from build123d import *

# Parameters (mm, degrees)
BOSS_EXTRUDE1_DEPTH = 16
SKETCH2_R           = 4
CUT_EXTRUDE1_DEPTH  = 40
SKETCH3_W           = 26
SKETCH3_H           = 4
CUT_EXTRUDE2_DEPTH  = 40
SKETCH4_R           = 1.25
CUT_EXTRUDE3_DEPTH  = 40


with BuildPart() as part:
    # Sketch1 → Boss-Extrude1 (new body)
    with BuildSketch(Plane.XY):
        Polygon((0, 0), (32, 0), (32, 12), (26, 18), (6, 18), (0, 12), align=None)
    extrude(amount=BOSS_EXTRUDE1_DEPTH)

    # Sketch2 → Cut-Extrude1 (cut, symmetric)
    with BuildSketch(Plane(origin=(0, 0, 0), x_dir=(1, 0, 0), z_dir=(0, 1, 0))):
        with Locations(Location((11, -8, 0), (0, 0, 270))):
            Circle(SKETCH2_R)
        with Locations(Location((21, -8, 0), (0, 0, 270))):
            Circle(SKETCH2_R)
    extrude(amount=CUT_EXTRUDE1_DEPTH, both=True, mode=Mode.SUBTRACT)

    # Sketch3 → Cut-Extrude2 (cut, symmetric)
    with BuildSketch(Plane.XY):
        with Locations((13, 6)):
            Rectangle(SKETCH3_W, SKETCH3_H)
    extrude(amount=CUT_EXTRUDE2_DEPTH, both=True, mode=Mode.SUBTRACT)

    # Sketch4 → Cut-Extrude3 (cut, symmetric)
    with BuildSketch(Plane.XY):
        with Locations((29, 11)):
            Circle(SKETCH4_R)
    extrude(amount=CUT_EXTRUDE3_DEPTH, both=True, mode=Mode.SUBTRACT)


solid = part.part
Geometry: final body of the model. Coordinates: model frame, mm. A direction names the side the tool comes from. Round coordinates to 2 decimals unless told otherwise and drop trailing zeros. Order: outer loops, then holes, each group sorted by start corner. A loop starts at its lowest first (then second) coordinate and runs counter-clockwise, first axis right, second up. Notation, with made-up numbers: (77.25, 42.25) -> (111.25, 42.25) arc R18 ccw to (111.25, 65.25) -> close; hole circle Ø5 at (85, 35). An arc over 180 degrees is marked (long way). Put each result on its own line as item: value. Start each with the question number.
Q1. Line query: probe 1 along X at (y, z) = (2.8, 8); probe 2 along Y at (x, z) = (25.5, 13.5); probe 3 along Y at (x, z) = (29, 10.5). Output: solid intervals per line, ascending.
Q2. First-contact query: pin 1 (1.5 mm diameter, centred on x = 29, y = 11, fed in from +Z). Flat tip, straight axial feed; report the tip coordinate or a pass-through.
Q3. Section B-B on z = 8. Return the cut outline in (x, y), and give its area (3 significant figures).
Q4. Section D-D on x = 29. Return the cut outline in (y, z).
Q5. Section A-A on y = 11. Return the cut outline in (x, z), and give its area (3 significant figures).
Q6. Reachability of faces 5 (the flat face through (0, 2, 8)), 6 (the flat face through (26, 6, 8)) from +Z, -Z, +X, -X, +Y, -Y: full face, straight path, thin tool, end or side. Return the list, or none.
Q7. Section C-C on x = 21. Return the cut outline in (y, z).
Q8. Pull-direction query (Y, two-part tool) for faces 1 (the flat face through (13, 8, 12)), 2 (the flat face through (13, 4, 12)), 3 (the flat face through (16, 0, 8)), 4 (the cylindrical face through (24.966, 2.028, 7.479)); classes: +Y half, -Y half, draft (parallel to the pull), parting line (faces both ways), or undercut.
Ans:
1. probe 1: x = 0 to 7, 15 to 17, 25 to 32
1. probe 2: y = 0 to 4, 8 to 18
1. probe 3: y = 0 to 9.75, 12.25 to 15
2. pin 1: passes through
3. outline: (0, 0) -> (7, 0) -> (7, 4) -> (0, 4) -> close; (0, 8) -> (7, 8) -> (7, 18) -> (6, 18) -> (0, 12) -> close; (15, 0) -> (17, 0) -> (17, 4) -> (15, 4) -> close; (15, 8) -> (17, 8) -> (17, 18) -> (15, 18) -> close; (25, 0) -> (32, 0) -> (32, 12) -> (26, 18) -> (25, 18) -> (25, 8) -> (26, 8) -> (26, 4) -> (25, 4) -> close; hole circle Ø2.5 at (29, 11)
3. area: 207 mm2
4. outline: (0, 0) -> (9.75, 0) -> (9.75, 16) -> (0, 16) -> close; (12.25, 0) -> (15, 0) -> (15, 16) -> (12.25, 16) -> close
5. outline: (0, 0) -> (27.75, 0) -> (27.75, 16) -> (0, 16) -> close; (30.25, 0) -> (32, 0) -> (32, 16) -> (30.25, 16) -> close; hole circle Ø8 at (11, 8); hole circle Ø8 at (21, 8)
5. area: 371 mm2
6. face 5: +Z, -Z, -X, +Y, -Y
6. face 6: +Z, -Z, -X
7. outline: (0, 0) -> (4, 0) -> (4, 4) -> (0, 4) -> close; (0, 12) -> (4, 12) -> (4, 16) -> (0, 16) -> close; (8, 0) -> (18, 0) -> (18, 4) -> (8, 4) -> close; (8, 12) -> (18, 12) -> (18, 16) -> (8, 16) -> close
8. face 1: undercut
8. face 2: undercut
8. face 3: -Y half
8. face 4: draft
